For this review, take the finished solid that the model builds, in its own axes (mm). Face numbers are marked on the shaded views. A direction names the side the tool comes from. Give positions to 0.01 mm unless a question says otherwise; leave off trailing zeros. Write each loop counter-clockwise with the first axis right and the second up, starting at its lowest first coordinate (ties: lowest second). Pieces come first, ordered by that corner, then holes.
1) We need section B-B on z = 5. Give the boundary of the cut face in (x, y).
2) We need section C-C on y = 10. Give the boundary of the cut face in (x, z).
3) For P1, Ø4, axis at y = 10, z = 5, coming from the +X side; P2, Ø5, axis at x = 5.5, y = 40.5, coming from the -Z side; P3, Ø5, axis at y = 10, z = 5.5, coming from the +X side; P4, Ø4, axis at x = 5, z = 7.5, coming from the -Y side, all flat-tipped, find the tip position at first contact; note any pin that passes through.
4) We need section D-D on x = 26.25. Give the boundary of the cut face in (y, z).
5) Wall thickness on line 1 along Y through (x, z) = (15.5, 4.5); line 2 along Y through (x, z) = (14.5, 5); line 3 along X through (y, z) = (7.5, 1.5): over which ranges is each line inside the solid? List them lowest first.
6) Machinability: for the marked faces 1 and 2, which of the approach directions +Z, -Z, +X, -X, +Y, -Y give a long, thin tool a straight path to every point of the face, cutting with its end or side? Answer none if there is none.
7) We need section A-A on x = 15. Give the boundary of the cut face in (y, z), and give its area (3 significant figures).
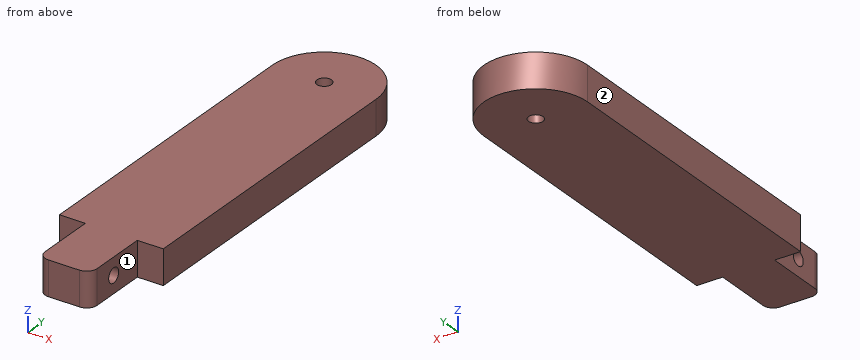
from build123d import *

# Parameters (mm, degrees)
SKETCH_1_W          = 30
SKETCH_1_H          = 125
EXTRUDE_1_DEPTH     = 10
SKETCH_2_W          = 7.5
SKETCH_2_H          = 20
CUT_EXTRUDE_1_DEPTH = 10
FILLET_1_R          = 3
SKETCH_3_R          = 2.1
CUT_EXTRUDE_2_DEPTH = 129.937969582
FILLET_2_RADIUS     = 15
FILLET_2_LENGTH     = 10
SKETCH_4_R          = 2.1
CUT_EXTRUDE_3_DEPTH = 129.937969582


with BuildPart() as part:
    # 草图1 → 凸台-拉伸1 (new body)
    with BuildSketch(Plane.XY):
        with Locations((15, 62.5)):
            Rectangle(SKETCH_1_W, SKETCH_1_H)
    extrude(amount=EXTRUDE_1_DEPTH)

    # 草图2 → 切除-拉伸1 (cut)
    with BuildSketch(Plane.XY.offset(10)):
        with Locations((3.75, 10)):
            Rectangle(SKETCH_2_W, SKETCH_2_H)
        with Locations((26.25, 10)):
            Rectangle(SKETCH_2_W, SKETCH_2_H)
    extrude(amount=-CUT_EXTRUDE_1_DEPTH, mode=Mode.SUBTRACT)

    # 圆角1
    fillet_1_edges = [part.edges().sort_by_distance(p)[0] for p in [
        (7.5, 0, 5),
        (22.5, 0, 5),
    ]]
    fillet(fillet_1_edges, radius=FILLET_1_R)

    # 草图3 → 切除-拉伸2 (cut, through all)
    with BuildSketch(Plane.ZY):
        with Locations((5, 10)):
            Circle(SKETCH_3_R)
    extrude(amount=-CUT_EXTRUDE_2_DEPTH, mode=Mode.SUBTRACT)

    # 圆角2: full round fillet: the end face becomes a half cylinder, R = half its width
    fillet_2_face = Plane((15, 125, 5), x_dir=(0, 0, 1), z_dir=(0, 1, 0))  # on the end face: x along it, z out of the body
    fillet_2_slab = fillet_2_face.offset(-FILLET_2_RADIUS / 2) * Box(FILLET_2_LENGTH, 2 * FILLET_2_RADIUS, FILLET_2_RADIUS, mode=Mode.PRIVATE)  # the body's end, R deep
    fillet_2_round = Plane((15, 110, 5), x_dir=(0, 1, 0), z_dir=(0, 0, 1)) * Cylinder(FILLET_2_RADIUS, FILLET_2_LENGTH, mode=Mode.PRIVATE)  # its axis R under the face
    add(fillet_2_slab - fillet_2_round, mode=Mode.SUBTRACT)

    # 草图4 → 切除-拉伸3 (cut, through all)
    with BuildSketch(Plane(origin=(0, 0, 0), x_dir=(-1, 0, 0), z_dir=(0, 0, -1))):
        with Locations((-15, 110)):
            Circle(SKETCH_4_R)
    extrude(amount=-CUT_EXTRUDE_3_DEPTH, mode=Mode.SUBTRACT)


solid = part.part
Results list:
1. outline: (0, 20) - (7.5, 20) - (7.5, 12.1) - (22.5, 12.1) - (22.5, 20) - (30, 20) - (30, 110) arc R15 ccw to (0, 110) - close; (7.5, 3) arc R3 ccw to (10.5, 0) - (19.5, 0) arc R3 ccw to (22.5, 3) - (22.5, 7.9) - (7.5, 7.9) - close; hole circle Ø4.2 at (15, 110)
2. outline: (7.5, 0) - (22.5, 0) - (22.5, 2.9) - (7.5, 2.9) - close; (7.5, 7.1) - (22.5, 7.1) - (22.5, 10) - (7.5, 10) - close
3. P1: passes through
3. P2: stops at z = 0
3. P3: stops at x = 22.5
3. P4: stops at y = 20
4. outline: (20, 0) - (119.92, 0) - (119.92, 10) - (20, 10) - close
5. line 1: y = 0 to 7.96, 12.04 to 107.96, 112.04 to 124.99
5. line 2: y = 0 to 7.9, 12.1 to 107.96, 112.04 to 124.99
5. line 3: x = 7.5 to 22.5
6. face 1: +Z, -Z, +X, -Y
6. face 2: +Z, -Z, -X, +Y, -Y
7. outline: (0, 0) - (107.9, 0) - (107.9, 10) - (0, 10) - close; (112.1, 0) - (125, 0) - (125, 10) - (112.1, 10) - close; hole circle Ø4.2 at (10, 5)
7. area: 1,190 mm2
